Could you check a few things on this model? Use its own coordinates, in mm. A direction names the side the tool comes from. Give positions to 0.01 mm unless a question says otherwise; leave off trailing zeros. Write each loop counter-clockwise with the first axis right and the second up, starting at its lowest first coordinate (ties: lowest second). Pieces come first, ordered by that corner, then holes. Notation, with made-up numbers: M 62,26 L 75,26 A23 ccw 75,43 Z; hole C 83.5,88 d1. An arc over 180 degrees is marked long. Use one line per item in the form item = value.
from build123d import *

# Parameters (mm, degrees)
F1_DEPTH = 12.7
F2_SIZE  = 25.39999
F3_DEPTH = 71.8420489686
F4_W     = 203.2
F4_H     = 70.0369336182
F4_H_2   = 71.8420560396
F4_H_3   = 35.9210103421
F5_DEPTH = 35.9156


# Not quite as in the source:
# - a fillet or chamfer is up to 0.001 mm smaller than in the source, because OpenCascade refuses the exact size


with BuildPart() as f1:
    # F0 (on Top) → F1 (new body, symmetric)
    with BuildSketch(Plane.XY):
        with BuildLine():
            Line((0, 76.2), (0, 0))
            Line((0, 0), (127, 0))
            Line((127, 0), (127, 203.2))
            Line((127, 203.2), (0, 203.2))
            Line((0, 203.2), (0, 127))
            Line((0, 127), (50.8, 127))
            ThreePointArc((50.8, 127), (76.2, 101.6), (50.8, 76.2))
            Line((50.8, 76.2), (0, 76.2))
        make_face()
    extrude(amount=F1_DEPTH, both=True)

    # F2 (size 25.4 in the source; OpenCascade refuses exactly that, so slightly less here)
    f2_edges = [f1.edges().sort_by_distance(p)[0] for p in [
        (127, 101.6, 12.7),
    ]]
    chamfer(f2_edges, length=F2_SIZE)

    # F3 (add): a face of the model
    f3_faces = [f1.faces().sort_by_distance(p)[0] for p in [
        (114.300005, 101.6, 5e-06),
    ]]
    extrude(f3_faces, amount=F3_DEPTH)

    # F4 (on face) → F5 (join)
    with BuildSketch(Plane(origin=(107.95, 0, 107.95), x_dir=(0, 1, 0), z_dir=(0.7071067812, 0, 0.7071067812))):
        with Locations((101.6, -27.8433331094)):
            Rectangle(F4_W, F4_H)
        with BuildLine():
            ThreePointArc((50.8, -30.9248663003), (38.1, -18.2248663003), (50.8, -5.5248663003))
            Line((50.8, -5.5248663003), (152.4, -5.5248663003))
            ThreePointArc((152.4, -5.5248663003), (165.1, -18.2248663003), (152.4, -30.9248663003))
            Line((152.4, -30.9248663003), (50.8, -30.9248663003))
        make_face(mode=Mode.SUBTRACT)
        with Locations((101.6, -134.7038382805)):
            Rectangle(F4_W, F4_H_2)
        with BuildLine():
            ThreePointArc((50.8, -157.9248663003), (38.1, -145.2248663003), (50.8, -132.5248663003))
            Line((50.8, -132.5248663003), (152.4, -132.5248663003))
            ThreePointArc((152.4, -132.5248663003), (165.1, -145.2248663003), (152.4, -157.9248663003))
            Line((152.4, -157.9248663003), (50.8, -157.9248663003))
        make_face(mode=Mode.SUBTRACT)
        with Locations((101.6, -80.8223050896)):
            Rectangle(F4_W, F4_H_3)
    extrude(amount=F5_DEPTH)


solid = f1.part
1) I want a section at B-B, the plane x = 106. Please give me the cut outline in (y, z).
Checked values:
outline = M 0,-12.7 L 203.2,-12.7 L 203.2,17.1 L 0,17.1 Z; M 0,109.9 L 203.2,109.9 L 203.2,116.15 L 0,116.15 Z
2) Thinking about a two-plate mould opening in X: for faces 4 (the flat face through (241.1, 100.2, -0.2)), 5 (the flat face through (132.8, 100.2, 83.1)), 6 (the flat face through (232.14, 102.31, 8.8)), which applies, released by +X, released by -X, zero draft, split by the parting line, or undercut?
Checked values:
face_4 = released by +X
face_5 = released by -X
face_6 = undercut
3) If I drill on L1, parallel to Z at x = 221, y = 51; L2, parallel to X at y = 70.5, z = 15.5; L3, parallel to Y at x = 128.5, z = 94, over which ranges is the centre line in solid material (lowest first)?
Checked values:
L1 = -5.1 to -2.34, 33.58 to 45.69
L2 = 104.4 to 155.2, 200.4 to 202.92, 238.84 to 251.19
L3 = 0 to 39.7, 163.5 to 203.2
4) For faces 1 (the flat face through (197.2, 100.2, 18.7)), 2 (the flat face through (142.337, 102.311, 98.603)), 3 (the flat face through (26, 76.2, 0)), which set-ups out of +Z, -Z, +X, -X, +Y, -Y let a thin tool reach every point of the face, with its end or its side?
Checked values:
face_1 = -Z, +Y, -Y
face_2 = none
face_3 = +Z, -Z, -X
5) For pin 1 Ø6 at (x, y) = (162, 176.5) entering from +Z; pin 2 Ø1.5 at (y, z) = (85.5, 53) entering from +X; pin 3 Ø4 at (y, z) = (153, 81.5) entering from -X, each with a flat end and sliding along its axis, tell me the tip position at first contact or that it passes through.
Checked values:
pin_1 = 107.69
pin_2 = 214.44
pin_3 = 132.4
6) I want a section at A-A, the plane y = 101.6. Count the separate pieces of the cut face and the enclosed holes in it, plus the area to 3 significant figures.
Checked values:
separate_pieces = 3
enclosed_holes = 0
area = 8,110 mm2
7) I want a section at D-D, the plane x = 66. Please give me the cut outline in (y, z), plus the area to 3 significant figures.
Checked values:
outline = M 0,-12.7 L 81.25,-12.7 L 81.25,12.7 L 0,12.7 Z; M 121.95,-12.7 L 203.2,-12.7 L 203.2,12.7 L 121.95,12.7 Z
area = 4,130 mm2
